Check sheet for the modelled part. Datum: model origin and axes. Units: mm. A direction names the side the tool comes from. Coordinates: 2 decimals unless noted, no trailing zeros. Loops run counter-clockwise (first coordinate to the right, second up) from the corner with the lowest first, then second, coordinate; pieces in that order, holes last.
```python
from build123d import *

# Parameters (mm, degrees)
SKETCH1_R             = 7.5
BOSS_EXTRUDE1_DEPTH   = 15
SKETCH2_R             = 2.45
BOSS_EXTRUDE2_DEPTH   = 6
SKETCH3_W             = 10.5
SKETCH3_H             = 5
SKETCH3_W_2           = 5
SKETCH3_H_2           = 10.5
BOSS_EXTRUDE3_DEPTH   = 2
FILLET1_R             = 2
F_2_0MM_DOWEL_HOLE1_D = 2
FILLET2_R             = 1


with BuildPart() as part:
    # Sketch1 → Boss-Extrude1 (new body)
    with BuildSketch(Plane(origin=(0, 0, 0), x_dir=(1, 0, 0), z_dir=(0, 1, 0))):
        Circle(SKETCH1_R)
    extrude(amount=BOSS_EXTRUDE1_DEPTH)

    # Sketch2 → Boss-Extrude2 (add)
    with BuildSketch(Plane(origin=(0, 15, 0), x_dir=(1, 0, 0), z_dir=(0, 1, 0))):
        Circle(SKETCH2_R)
    extrude(amount=BOSS_EXTRUDE2_DEPTH)

    # Sketch3 → Boss-Extrude3 (add)
    with BuildSketch(Plane(origin=(0, 0, 0), x_dir=(1, 0, 0), z_dir=(0, 1, 0))):
        with Locations((-7.75, 0)):
            Rectangle(SKETCH3_W, SKETCH3_H)
        with Locations((0, -7.75)):
            Rectangle(SKETCH3_W_2, SKETCH3_H_2)
        with Locations((7.75, 0)):
            Rectangle(SKETCH3_W, SKETCH3_H)
        with Locations((0, 7.75)):
            Rectangle(SKETCH3_W_2, SKETCH3_H_2)
    extrude(amount=BOSS_EXTRUDE3_DEPTH)

    # Fillet1
    fillet1_edges = [part.edges().sort_by_distance(p)[0] for p in [
        (-7.5, 2, 0),
        (-7.071067812, 1, 2.5),
        (-7.071067812, 1, -2.5),
        (0, 2, 7.5),
        (-2.5, 1, 7.071067812),
        (2.5, 1, 7.071067812),
        (7.391989197, 2, -1.26826484),
        (7.071067812, 1, 2.5),
        (7.071067812, 1, -2.5),
        (0, 2, -7.5),
        (-2.5, 1, -7.071067812),
        (2.5, 1, -7.071067812),
    ]]
    fillet(fillet1_edges, radius=FILLET1_R)

    # Ø2.0mm Dowel Hole1 (through all)
    with Locations(Plane(origin=(-11.3, 2, 0), x_dir=(0, 0, 1), z_dir=(0, 1, 0))):
        with Locations((0, 0), (-11.3, 11.3), (0, 22.6), (11.3, 11.3)):
            Hole(F_2_0MM_DOWEL_HOLE1_D / 2)

    # Fillet2
    fillet2_edges = [part.edges().sort_by_distance(p)[0] for p in [
        (-2.45, 21, 0),
    ]]
    fillet(fillet2_edges, radius=FILLET2_R)


solid = part.part
```
1) Section check C-C on x = 0. Enter the section's corners in (y, z), plus the area to 3 significant figures.
Answer sheet:
outline: (0, -13) - (2, -13) - (2, -12.3) - (0, -12.3) - close; (0, -10.3) - (2, -10.3) - (2, -9.5) arc R2 cw to (4, -7.5) - (15, -7.5) - (15, -2.45) - (20, -2.45) arc R1 ccw to (21, -1.45) - (21, 1.45) arc R1 ccw to (20, 2.45) - (15, 2.45) - (15, 7.5) - (4, 7.5) arc R2 cw to (2, 9.5) - (2, 10.3) - (0, 10.3) - close; (0, 12.3) - (2, 12.3) - (2, 13) - (0, 13) - close
area: 270 mm2
2) Set-up check for faces 1 (the flat face through (-2.5, 1, 11)), 2 (the flat face through (11, 1, -2.5)), 3 (the flat face through (-10, 2, 0)), 4 (the flat face through (-2.5, 1, -11)): record each of +Z, -Z, +X, -X, +Y, -Y from which the full face is reachable in a straight line by a thin tool's end or side.
Answer sheet:
face 1: +Z, -X, +Y, -Y
face 2: -Z, +X, +Y, -Y
face 3: +Z, -Z, -X, +Y
face 4: -Z, -X, +Y, -Y
3) Section check A-A on z = 0. Enter the section's corners in (x, y), plus the area to 3 significant figures.
Answer sheet:
outline: (-13, 0) - (-12.3, 0) - (-12.3, 2) - (-13, 2) - close; (-10.3, 0) - (10.3, 0) - (10.3, 2) - (9.5, 2) arc R2 cw to (7.5, 4) - (7.5, 15) - (2.45, 15) - (2.45, 20) arc R1 ccw to (1.45, 21) - (-1.45, 21) arc R1 ccw to (-2.45, 20) - (-2.45, 15) - (-7.5, 15) - (-7.5, 4) arc R2 cw to (-9.5, 2) - (-10.3, 2) - close; (12.3, 0) - (13, 0) - (13, 2) - (12.3, 2) - close
area: 270 mm2
4) Mould release check, pull along Z, two halves, no side actions. Record for faces 5 (the cylindrical face through (0.3, 0.986, -12.254)), 6 (the cylindrical face through (2.93, 1.53, 7.13)), 7 (the flat face through (0, 1, -13)): +Z half, -Z half, draft (parallel to the pull), parting line (faces both ways), or undercut.
Answer sheet:
face 5: undercut
face 6: +Z half
face 7: -Z half
5) Section check D-D on z = 11.3. Enter the section's corners in (x, y), plus the area to 3 significant figures.
Answer sheet:
outline: (-2.5, 0) - (-1, 0) - (-1, 2) - (-2.5, 2) - close; (1, 0) - (2.5, 0) - (2.5, 2) - (1, 2) - close
area: 6.00 mm2
6) Scan lines: line 1 (X direction, y = 1.4, z = 11.3); line 2 (X direction, y = 1.15, z = 0); line 3 (Y direction, x = -9.25, z = 1.25). Record each from-to range of solid material in increasing order.
Answer sheet:
line 1: x = -2.5 to -1, 1 to 2.5
line 2: x = -13 to -12.3, -10.3 to 10.3, 12.3 to 13
line 3: y = 0 to 2.01
7) Depth check by flat-ended pin: pin 1 (6 mm diameter, centred on x = -10, z = 4.5, fed in from -Y); pin 2 (1.9 mm diameter, centred on x = -0.5, z = -10.5, fed in from +Y); pin 3 (1.7 mm diameter, centred on x = -10, y = 1.5, fed in from +Z); pin 4 (12 mm diameter, centred on y = 16.5, z = -6.5, fed in from +X). Enter the tip coordinate at first touch or a pass-through.
Answer sheet:
pin 1: stops at y = 0
pin 2: stops at y = 2
pin 3: stops at z = 2.5
pin 4: stops at x = 7.47
8) Section check B-B on x = 11.3. Enter the section's corners in (y, z), plus the area to 3 significant figures.
Answer sheet:
outline: (0, -2.5) - (2, -2.5) - (2, -1) - (0, -1) - close; (0, 1) - (2, 1) - (2, 2.5) - (0, 2.5) - close
area: 6.00 mm2
